```python
from build123d import *

# Parameters (mm, degrees)
BOSS_EXTRUDE1_DEPTH      = 30
BOSS_EXTRUDE1_DEPTH_BACK = 20
BOSS_EXTRUDE2_DEPTH      = 10
SKETCH2_R                = 5
CUT_EXTRUDE1_DEPTH       = 30
CUT_EXTRUDE3_START       = -30
SKETCH3_R                = 5
CUT_EXTRUDE3_DEPTH       = 30
CUT_EXTRUDE5_DEPTH       = 330.165611813
CUT_EXTRUDE7_DEPTH       = 20
CUT_EXTRUDE8_START       = -20
CUT_EXTRUDE8_DEPTH       = 20
CHAMFER7_SIZE            = 15
CUT_EXTRUDE6_DEPTH       = 8.5
SKETCH2_4_R              = 5
CUT_EXTRUDE2_DEPTH       = 8.5


with BuildPart() as part:
    # Sketch1 → Boss-Extrude1 (new, two sides: drawn at the far end of the back side and taken through both)
    with BuildSketch(Plane(origin=(0, 0, 0), x_dir=(1, 0, 0), z_dir=(0, 1, 0)).offset(-BOSS_EXTRUDE1_DEPTH_BACK)):
        with BuildLine():
            Line((30, 0), (190, 0))
            ThreePointArc((190, 0), (211.213203436, 8.786796564), (220, 30))
            Line((220, 30), (220, 200))
            ThreePointArc((220, 200), (211.213203436, 221.213203436), (190, 230))
            Line((190, 230), (30, 230))
            ThreePointArc((30, 230), (8.786796564, 221.213203436), (0, 200))
            Line((0, 200), (0, 30))
            ThreePointArc((0, 30), (8.786796564, 8.786796564), (30, 0))
        make_face()
    extrude(amount=BOSS_EXTRUDE1_DEPTH + BOSS_EXTRUDE1_DEPTH_BACK)

    # Sketch1<3> → Boss-Extrude2 (add)
    with BuildSketch(Plane(origin=(0, 0, 0), x_dir=(1, 0, 0), z_dir=(0, 1, 0))):
        with BuildLine():
            Line((-5, 30), (-5, 200))
            ThreePointArc((-5, 200), (5.251262658, 224.748737342), (30, 235))
            Line((30, 235), (190, 235))
            ThreePointArc((190, 235), (214.748737342, 224.748737342), (225, 200))
            Line((225, 200), (225, 30))
            ThreePointArc((225, 30), (214.748737342, 5.251262658), (190, -5))
            Line((190, -5), (30, -5))
            ThreePointArc((30, -5), (5.251262658, 5.251262658), (-5, 30))
        make_face()
        with BuildLine():
            Line((30, 0), (190, 0))
            ThreePointArc((190, 0), (211.213203436, 8.786796564), (220, 30))
            Line((220, 30), (220, 200))
            ThreePointArc((220, 200), (211.213203436, 221.213203436), (190, 230))
            Line((190, 230), (30, 230))
            ThreePointArc((30, 230), (8.786796564, 221.213203436), (0, 200))
            Line((0, 200), (0, 30))
            ThreePointArc((0, 30), (8.786796564, 8.786796564), (30, 0))
        make_face(mode=Mode.SUBTRACT)
    extrude(amount=BOSS_EXTRUDE2_DEPTH)

    # Sketch2 → Cut-Extrude1 (cut)
    with BuildSketch(Plane(origin=(0, 0, -230), x_dir=(-1, 0, 0), z_dir=(0, 0, -1))):
        with Locations((-150, 20)):
            Circle(SKETCH2_R)
        with Locations(Location((-70, 20, 0), (0, 0, 180))):
            Circle(SKETCH2_R)
        with Locations((-70, -10)):
            Circle(SKETCH2_R)
        with Locations(Location((-150, -10, 0), (0, 0, 180))):
            Circle(SKETCH2_R)
    extrude(amount=-CUT_EXTRUDE1_DEPTH, mode=Mode.SUBTRACT)

    # Sketch3 → Cut-Extrude3 (cut)
    with BuildSketch(Plane.XY.offset(CUT_EXTRUDE3_START)):
        with Locations((70, 20)):
            Circle(SKETCH3_R)
        with Locations(Location((150, 20, 0), (0, 0, 180))):
            Circle(SKETCH3_R)
        with Locations((150, -10)):
            Circle(SKETCH3_R)
        with Locations(Location((70, -10, 0), (0, 0, 180))):
            Circle(SKETCH3_R)
    extrude(amount=CUT_EXTRUDE3_DEPTH, mode=Mode.SUBTRACT)

    # Sketch4 → Cut-Extrude5 (cut, through all)
    with BuildSketch(Plane(origin=(0, 30, 0), x_dir=(1, 0, 0), z_dir=(0, 1, 0))):
        with BuildLine():
            Line((135, 165), (85, 165))
            ThreePointArc((85, 165), (75, 175), (85, 185))
            Line((85, 185), (135, 185))
            ThreePointArc((135, 185), (145, 175), (135, 165))
        make_face()
    extrude(amount=-CUT_EXTRUDE5_DEPTH, mode=Mode.SUBTRACT)

    # Sketch7 → Cut-Extrude7 (cut)
    with BuildSketch(Plane(origin=(0, 30, 0), x_dir=(1, 0, 0), z_dir=(0, 1, 0))):
        with BuildLine():
            Line((215, 30), (215, 200))
            ThreePointArc((215, 200), (207.67766953, 217.67766953), (190, 225))
            Line((190, 225), (30, 225))
            ThreePointArc((30, 225), (12.32233047, 217.67766953), (5, 200))
            Line((5, 200), (5, 30))
            ThreePointArc((5, 30), (12.32233047, 12.32233047), (30, 5))
            Line((30, 5), (190, 5))
            ThreePointArc((190, 5), (207.67766953, 12.32233047), (215, 30))
        make_face()
    extrude(amount=-CUT_EXTRUDE7_DEPTH, mode=Mode.SUBTRACT)

    # Sketch9 → Cut-Extrude8 (cut)
    with BuildSketch(Plane.XZ.offset(20).offset(CUT_EXTRUDE8_START)):
        with BuildLine():
            Line((190, -5), (30, -5))
            ThreePointArc((30, -5), (12.32233047, -12.32233047), (5, -30))
            Line((5, -30), (5, -200))
            ThreePointArc((5, -200), (12.32233047, -217.67766953), (30, -225))
            Line((30, -225), (190, -225))
            ThreePointArc((190, -225), (207.67766953, -217.67766953), (215, -200))
            Line((215, -200), (215, -30))
            ThreePointArc((215, -30), (207.67766953, -12.32233047), (190, -5))
        make_face()
    extrude(amount=CUT_EXTRUDE8_DEPTH, mode=Mode.SUBTRACT)

    # Chamfer7
    # the kernel refuses this chamfer: 15 mm, written as the material it adds along each edge
    with BuildSketch(Plane(origin=(190, 10, -225), x_dir=(0, 0.9996219169112968, -0.02749587661058586), z_dir=(-1, 0, 0))) as chamfer7_piece_1_section:
        Polygon((CHAMFER7_SIZE * 0.999621916911, -CHAMFER7_SIZE * 0.0274958766106), (-CHAMFER7_SIZE * 0.0274958766106, -CHAMFER7_SIZE * 0.999621916911), (0, 0), align=None)
    chamfer7_piece_1 = extrude(amount=160, mode=Mode.PRIVATE)
    chamfer7_piece_1 = chamfer7_piece_1 - Plane(origin=(150, 20, -219.960339284), x_dir=(-1, 0, 0), z_dir=(0, 0, -1)) * Cylinder(5, 380, mode=Mode.PRIVATE)
    chamfer7_piece_1 = chamfer7_piece_1 - Plane(origin=(70, 20, -219.960339284), x_dir=(1, 0, 0), z_dir=(0, 0, -1)) * Cylinder(5, 380, mode=Mode.PRIVATE)
    add(chamfer7_piece_1)
    with BuildSketch(Plane(origin=(30, 10, -5), x_dir=(0, 0.9996219169112968, 0.02749587661058638), z_dir=(1, 0, 0))) as chamfer7_piece_2_section:
        Polygon((CHAMFER7_SIZE * 0.999621916911, -CHAMFER7_SIZE * 0.0274958766106), (-CHAMFER7_SIZE * 0.0274958766106, -CHAMFER7_SIZE * 0.999621916911), (0, 0), align=None)
    chamfer7_piece_2 = extrude(amount=160, mode=Mode.PRIVATE)
    chamfer7_piece_2 = chamfer7_piece_2 - Plane(origin=(70, 20, -10.039660716), x_dir=(1, 0, 0), z_dir=(0, 0, -1)) * Cylinder(5, 380, mode=Mode.PRIVATE)
    chamfer7_piece_2 = chamfer7_piece_2 - Plane(origin=(150, 20, -10.039660716), x_dir=(-1, 0, 0), z_dir=(0, 0, -1)) * Cylinder(5, 380, mode=Mode.PRIVATE)
    add(chamfer7_piece_2)
    with BuildSketch(Plane(origin=(190, 10, -30), x_dir=(0, 0, 1), z_dir=(-1, 0, 0))) as chamfer7_piece_3:
        Polygon((25, CHAMFER7_SIZE), (25 - CHAMFER7_SIZE, 0), (25, 0), align=None)
    revolve(axis=Axis((190, 10, -30), (0, 1, 0)), revolution_arc=90)
    with BuildSketch(Plane(origin=(30, 10, -30), x_dir=(-1, 0, 0), z_dir=(0, 0, -1))) as chamfer7_piece_4:
        Polygon((25, CHAMFER7_SIZE), (25 - CHAMFER7_SIZE, 0), (25, 0), align=None)
    revolve(axis=Axis((30, 10, -30), (0, 1, 0)), revolution_arc=90)
    with BuildSketch(Plane(origin=(5, 10, -200), x_dir=(-0.02749587661058638, 0.9996219169112968, 0), z_dir=(0, 0, 1)), Plane(origin=(215, 10, -30), x_dir=(0.02749587661058586, 0.9996219169112968, 0), z_dir=(0, 0, -1))) as chamfer7_piece_5:
        Polygon((CHAMFER7_SIZE * 0.999621916911, -CHAMFER7_SIZE * 0.0274958766106), (-CHAMFER7_SIZE * 0.0274958766106, -CHAMFER7_SIZE * 0.999621916911), (0, 0), align=None)
    extrude(amount=170)
    with BuildSketch(Plane(origin=(30, 10, -200), x_dir=(0, 0, -1), z_dir=(1, 0, 0))) as chamfer7_piece_6:
        Polygon((25, CHAMFER7_SIZE), (25 - CHAMFER7_SIZE, 0), (25, 0), align=None)
    revolve(axis=Axis((30, 10, -200), (0, 1, 0)), revolution_arc=90)
    with BuildSketch(Plane(origin=(190, 10, -200), x_dir=(1, 0, 0), z_dir=(0, 0, 1))) as chamfer7_piece_7:
        Polygon((25, CHAMFER7_SIZE), (25 - CHAMFER7_SIZE, 0), (25, 0), align=None)
    revolve(axis=Axis((190, 10, -200), (0, 1, 0)), revolution_arc=90)
    with BuildSketch(Plane(origin=(30, 0, -225), x_dir=(0, 0.027495876610586382, 0.9996219169112968), z_dir=(1, 0, 0))) as chamfer7_piece_8_section:
        Polygon((CHAMFER7_SIZE * 0.999621916911, CHAMFER7_SIZE * 0.0274958766106), (-CHAMFER7_SIZE * 0.0274958766106, CHAMFER7_SIZE * 0.999621916911), (0, 0), align=None)
    chamfer7_piece_8 = extrude(amount=160, mode=Mode.PRIVATE)
    chamfer7_piece_8 = chamfer7_piece_8 - Plane(origin=(150, -10, -219.960344511), x_dir=(1, 0, 0), z_dir=(0, 0, -1)) * Cylinder(5, 380, mode=Mode.PRIVATE)
    chamfer7_piece_8 = chamfer7_piece_8 - Plane(origin=(70, -10, -219.960344511), x_dir=(-1, 0, 0), z_dir=(0, 0, -1)) * Cylinder(5, 380, mode=Mode.PRIVATE)
    add(chamfer7_piece_8)
    with BuildSketch(Plane(origin=(190, 0, -5), x_dir=(0, 0.02749587661058637, -0.9996219169112968), z_dir=(-1, 0, 0))) as chamfer7_piece_9_section:
        Polygon((CHAMFER7_SIZE * 0.999621916911, CHAMFER7_SIZE * 0.0274958766106), (-CHAMFER7_SIZE * 0.0274958766106, CHAMFER7_SIZE * 0.999621916911), (0, 0), align=None)
    chamfer7_piece_9 = extrude(amount=160, mode=Mode.PRIVATE)
    chamfer7_piece_9 = chamfer7_piece_9 - Plane(origin=(150, -10, -10.039655489), x_dir=(1, 0, 0), z_dir=(0, 0, -1)) * Cylinder(5, 380, mode=Mode.PRIVATE)
    chamfer7_piece_9 = chamfer7_piece_9 - Plane(origin=(70, -10, -10.039655489), x_dir=(-1, 0, 0), z_dir=(0, 0, -1)) * Cylinder(5, 380, mode=Mode.PRIVATE)
    add(chamfer7_piece_9)
    with BuildSketch(Plane(origin=(30, 0, -30), x_dir=(0, 0, 1), z_dir=(1, 0, 0))) as chamfer7_piece_10:
        Polygon((25 - CHAMFER7_SIZE, 0), (25, CHAMFER7_SIZE), (25, 0), align=None)
    revolve(axis=Axis((30, 0, -30), (0, -1, 0)), revolution_arc=90)
    with BuildSketch(Plane(origin=(190, 0, -30), x_dir=(1, 0, 0), z_dir=(0, 0, -1))) as chamfer7_piece_11:
        Polygon((25 - CHAMFER7_SIZE, 0), (25, CHAMFER7_SIZE), (25, 0), align=None)
    revolve(axis=Axis((190, 0, -30), (0, -1, 0)), revolution_arc=90)
    with BuildSketch(Plane(origin=(215, 0, -200), x_dir=(-0.9996219169112966, 0.02749587661058638, 0), z_dir=(0, 0, 1)), Plane(origin=(5, 0, -30), x_dir=(0.9996219169112966, 0.027495876610586358, 0), z_dir=(0, 0, -1))) as chamfer7_piece_12:
        Polygon((CHAMFER7_SIZE * 0.999621916911, CHAMFER7_SIZE * 0.0274958766106), (-CHAMFER7_SIZE * 0.0274958766106, CHAMFER7_SIZE * 0.999621916911), (0, 0), align=None)
    extrude(amount=170)
    with BuildSketch(Plane(origin=(190, 0, -200), x_dir=(0, 0, -1), z_dir=(-1, 0, 0))) as chamfer7_piece_13:
        Polygon((25 - CHAMFER7_SIZE, 0), (25, CHAMFER7_SIZE), (25, 0), align=None)
    revolve(axis=Axis((190, 0, -200), (0, -1, 0)), revolution_arc=90)
    with BuildSketch(Plane(origin=(30, 0, -200), x_dir=(-1, 0, 0), z_dir=(0, 0, 1))) as chamfer7_piece_14:
        Polygon((25 - CHAMFER7_SIZE, 0), (25, CHAMFER7_SIZE), (25, 0), align=None)
    revolve(axis=Axis((30, 0, -200), (0, -1, 0)), revolution_arc=90)

    # Sketch6 → Cut-Extrude6 (cut)
    with BuildSketch(Plane.XY):
        Polygon((140.762833455, 19.910069191), (145.459299093, 11.955413708), (154.696465638, 12.045344517), (159.237166545, 20.089930809), (154.540700907, 28.044586292), (145.303534362, 27.954655483), align=None)
        Polygon((65.285101729, 27.94374393), (60.76306682, 19.888650286), (65.477965091, 11.944906356), (74.714898271, 12.05625607), (79.23693318, 20.111349714), (74.522034909, 28.055093644), align=None)
        Polygon((140.763314396, -9.869721899), (145.268833053, -17.934065329), (154.505518657, -18.064343431), (159.236685604, -10.130278101), (154.731166947, -2.065934671), (145.494481343, -1.935656569), align=None)
        Polygon((60.763314396, -9.869721899), (65.268833053, -17.934065329), (74.505518657, -18.064343431), (79.236685604, -10.130278101), (74.731166947, -2.065934671), (65.494481343, -1.935656569), align=None)
    extrude(amount=-CUT_EXTRUDE6_DEPTH, mode=Mode.SUBTRACT)

    # Sketch2<4> → Cut-Extrude2 (cut)
    # profile 1 of 4: a face of its own
    with BuildSketch(Plane(origin=(0, 0, -230), x_dir=(-1, 0, 0), z_dir=(0, 0, -1))):
        Polygon((-74.618802154, 12), (-79.237604307, 20), (-74.618802154, 28), (-65.381197846, 28), (-60.762395693, 20), (-65.381197846, 12), align=None)
        with Locations((-70, 20)):
            Circle(SKETCH2_4_R, mode=Mode.SUBTRACT)
    # profile 2 of 4: a face of its own
    with BuildSketch(Plane(origin=(0, 0, -230), x_dir=(-1, 0, 0), z_dir=(0, 0, -1))):
        Polygon((-140.762395693, 20), (-145.381197846, 28), (-154.618802154, 28), (-159.237604307, 20), (-154.618802154, 12), (-145.381197846, 12), align=None)
        with Locations((-150, 20)):
            Circle(SKETCH2_4_R, mode=Mode.SUBTRACT)
    # profile 3 of 4: a face of its own
    with BuildSketch(Plane(origin=(0, 0, -230), x_dir=(-1, 0, 0), z_dir=(0, 0, -1))):
        Polygon((-65.381197846, -2), (-74.618802154, -2), (-79.237604307, -10), (-74.618802154, -18), (-65.381197846, -18), (-60.762395693, -10), align=None)
        with Locations((-70, -10)):
            Circle(SKETCH2_4_R, mode=Mode.SUBTRACT)
    # profile 4 of 4: a face of its own
    with BuildSketch(Plane(origin=(0, 0, -230), x_dir=(-1, 0, 0), z_dir=(0, 0, -1))):
        Polygon((-145.381197846, -2), (-140.762395693, -10), (-145.381197846, -18), (-154.618802154, -18), (-159.237604307, -10), (-154.618802154, -2), align=None)
        with Locations((-150, -10)):
            Circle(SKETCH2_4_R, mode=Mode.SUBTRACT)
    extrude(amount=-CUT_EXTRUDE2_DEPTH, mode=Mode.SUBTRACT)


solid = part.part
```
CAD build for the part. Positions are in the model's coordinates, mm. A direction names the side the tool comes from. Round coordinates to 2 decimals unless told otherwise and drop trailing zeros. Order: outer loops, then holes, each group sorted by start corner. A loop starts at its lowest first (then second) coordinate and runs counter-clockwise, first axis right, second up.
Q1. Two-plate mould, pull along X, no slides. Class faces 5 (the flat face through (143.078, 15.988, -4.19)), 6 (the cylindrical face through (8.555, 19.86, -9.021)), 7 (the flat face through (111, -10, -230)), 8 (the flat face through (220, -10, -114)): pulls with the +X half, pulls with the -X half, needs draft (parallel to the pull), parting line crosses it, or undercut.
Q2. Wall check: L1, parallel to Z at x = 102.5, y = 26.5; L2, parallel to Y at x = 65.5, z = -34.5; L3, parallel to X at y = 20, z = -13. Give the ranges that are in metal, low to high.
Q3. Slice it at B-B (z = -175). Write the cut outline in (x, y), and give its area (3 significant figures).
Q4. Slice it at D-D (z = -134). Write the cut outline in (x, y), and give its area (3 significant figures).
Q5. Slice it at C-C (y = 5.5). Write the cut outline in (x, z).
Q6. Which spindle directions (+Z, -Z, +X, -X, +Y, -Y) get a long thin tool onto all of the face, cutting with end or side? Do faces 1 (the cylindrical face through (8.555, -10.14, -9.021)), 2 (the flat face through (109, 10, -116)), 3 (the flat face through (156.935, 16.011, -4.19)), 4 (the flat face through (62.591, 23.167, -226.754)). Say none if no direction does.
Q7. Drop flat-ended pins along their axis: pin 1 (11.5 mm diameter, centred on x = 150, y = -10, fed in from -Z); pin 2 (8 mm diameter, centred on y = -5, z = -172.5, fed in from -X); pin 3 (10.5 mm diameter, centred on x = 154, y = -7, fed in from +Z); pin 4 (6 mm diameter, centred on x = 150, y = 20, fed in from +Z). Give the stop position or say it passes through.
Q8. Slice it at A-A (x = 131). Write the cut outline in (y, z), and give its area (3 significant figures).
Results below:
1. face 5: undercut
1. face 6: pulls with the -X half
1. face 7: needs draft
1. face 8: pulls with the +X half
2. L1: z = -230 to -225, -5 to 0
2. L2: y = 0 to 10
2. L3: x = 5.28 to 19.46, 200.54 to 214.72
3. outline: (-5, 0) - (0, 0) - (0, -20) - (5, -20) - (5, -15) - (20, 0) - (75, 0) - (75, 10) - (20, 10) - (5, 25) - (5, 30) - (0, 30) - (0, 10) - (-5, 10) - close; (145, 0) - (200, 0) - (215, -15) - (215, -20) - (220, -20) - (220, 0) - (225, 0) - (225, 10) - (220, 10) - (220, 30) - (215, 30) - (215, 25) - (200, 10) - (145, 10) - close
3. area: 2,450 mm2
4. outline: (-5, 0) - (0, 0) - (0, -20) - (5, -20) - (5, -15) - (20, 0) - (200, 0) - (215, -15) - (215, -20) - (220, -20) - (220, 0) - (225, 0) - (225, 10) - (220, 10) - (220, 30) - (215, 30) - (215, 25) - (200, 10) - (20, 10) - (5, 25) - (5, 30) - (0, 30) - (0, 10) - (-5, 10) - close
4. area: 3,150 mm2
5. outline: (-5, -200) arc R35 ccw to (30, -235) - (190, -235) arc R35 ccw to (225, -200) - (225, -30) arc R35 ccw to (190, 5) - (30, 5) arc R35 ccw to (-5, -30) - close; hole (85, -185) - (135, -185) arc R10 ccw to (135, -165) - (85, -165) arc R10 ccw to start
6. face 1: +Z, -X, -Y
6. face 2: +Y
6. face 3: +Z
6. face 4: -Z
7. pin 1: stops at z = -221.5
7. pin 2: stops at x = 0
7. pin 3: stops at z = 0
7. pin 4: passes through
8. outline: (-20, -230) - (0, -230) - (0, -235) - (10, -235) - (10, -230) - (30, -230) - (30, -225) - (25, -225) - (10, -210) - (10, -185) - (0, -185) - (0, -210) - (-15, -225) - (-20, -225) - close; (-20, -5) - (-15, -5) - (0, -20) - (0, -165) - (10, -165) - (10, -20) - (25, -5) - (30, -5) - (30, 0) - (10, 0) - (10, 5) - (0, 5) - (0, 0) - (-20, 0) - close
8. area: 3,050 mm2
